Geometry check sheet. Reference: the model listing, model coordinates, mm. A direction names the side the tool comes from. Round coordinates to 2 decimals unless told otherwise and drop trailing zeros. Loops run counter-clockwise (first coordinate to the right, second up) from the corner with the lowest first, then second, coordinate; pieces in that order, holes last.
```python
from build123d import *

# Parameters (mm, degrees)
SKETCH_1_W      = 10
SKETCH_1_H      = 20
SKETCH_1_R      = 1.25
EXTRUDE_1_DEPTH = 1
FILLET_1_R      = 1
SKETCH_13_R     = 0.75


with BuildPart() as part:
    # 草图1 → 凸台-拉伸1 (new body)
    with BuildSketch(Plane.XY):
        with Locations((5, -10)):
            Rectangle(SKETCH_1_W, SKETCH_1_H)
        with Locations((5, -4)):
            Circle(SKETCH_1_R, mode=Mode.SUBTRACT)
        with Locations((5, -16)):
            Circle(SKETCH_1_R, mode=Mode.SUBTRACT)
    extrude(amount=EXTRUDE_1_DEPTH)

    # 圆角1
    fillet_1_edges = [part.edges().sort_by_distance(p)[0] for p in [
        (0, 0, 0.5),
        (10, 0, 0.5),
        (10, -20, 0.5),
        (0, -20, 0.5),
    ]]
    fillet(fillet_1_edges, radius=FILLET_1_R)

    # 扫描11: sweep along a path in 草图5
    with BuildLine(Plane(origin=(0, -10, 0), x_dir=(1, 0, 0), z_dir=(0, 1, 0))) as sweep_11_path:
        Line((1.3, 0), (1.3, 11.5))
        ThreePointArc((1.3, 11.5), (1.739339828, 12.560660172), (2.8, 13))
        Line((2.8, 13), (7.2, 13))
        ThreePointArc((7.2, 13), (8.260660172, 12.560660172), (8.7, 11.5))
        Line((8.7, 11.5), (8.7, 0))
    # 草图13 → 扫描11 (sweep)
    with BuildSketch(Plane(origin=(0, 0, 0), x_dir=(-1, 0, 0), z_dir=(0, 0, -1))):
        with Locations((-8.7, -10)):
            Circle(SKETCH_13_R)
    sweep(path=sweep_11_path.line)


solid = part.part
```
1) Sectioned sample at D-D, the plane z = -0.75. Record the cut outline in (x, y), then the cut area to 3 significant figures.
Report:
outline: circle Ø1.5 at (1.3, -10); circle Ø1.5 at (8.7, -10)
area: 3.53 mm2
2) Sectioned sample at C-C, the plane y = -10. Record the cut outline in (x, z).
Report:
outline: (0, 0) - (0.55, 0) - (0.55, -11.5) arc R2.25 ccw to (2.8, -13.75) - (7.2, -13.75) arc R2.25 ccw to (9.45, -11.5) - (9.45, 0) - (10, 0) - (10, 1) - (0, 1) - close; hole (2.05, -11.5) arc R0.75 ccw to (2.8, -12.25) - (7.2, -12.25) arc R0.75 ccw to (7.95, -11.5) - (7.95, 0) - (2.05, 0) - close
3) Sectioned sample at A-A, the plane y = -4. Record the cut outline in (x, z), then the cut area to 3 significant figures.
Report:
outline: (0, 0) - (3.75, 0) - (3.75, 1) - (0, 1) - close; (6.25, 0) - (10, 0) - (10, 1) - (6.25, 1) - close
area: 7.50 mm2
4) Mould release check, pull along Z, two halves, no side actions. Record for faces 1 (the face through (0.285, -19.699, 0.507)), 2 (the face through (5, -10, 1)), 3 (the face through (5.03, -10.51, -13.55)): +Z half, -Z half, draft (parallel to the pull), parting line (faces both ways), or undercut.
Report:
face 1: draft
face 2: +Z half
face 3: undercut
5) Sectioned sample at B-B, the plane x = 6. Record the cut outline in (y, z).
Report:
outline: (-20, 0) - (-16.75, 0) - (-16.75, 1) - (-20, 1) - close; (-15.25, 0) - (-4.75, 0) - (-4.75, 1) - (-15.25, 1) - close; circle Ø1.5 at (-10, -13); (-3.25, 0) - (0, 0) - (0, 1) - (-3.25, 1) - close
6) Scan lines: line 1 along Y through (x, z) = (5, 0.35); line 2 along Z through (x, y) = (2, -3.25); line 3 along Z through (x, y) = (7.75, -9.5). Record each from-to range of solid material in increasing order.
Report:
line 1: y = -20 to -17.25, -14.75 to -5.25, -2.75 to 0
line 2: z = 0 to 1
line 3: z = -13.48 to -12.26, 0 to 1
7) Access from +Z, -Z, +X, -X, +Y, -Y to the whole of each face (thin tool, end or side, straight path). Record for faces 4 (the face through (1.202, -10.744, -5.83)), 5 (the face through (9.699, -19.715, 0.507)).
Report:
face 4: none
face 5: +Z, -Z, +X, -Y
8) Gauge pin test, flat ends, axial feed: pin 1 (2 mm diameter, centred on x = 5, y = -4, fed in from -Z); pin 2 (3 mm diameter, centred on x = 5, y = -16, fed in from -Z); pin 3 (3 mm diameter, centred on y = -10.5, z = -5.5, fed in from +X). Record the tip position at first contact, or that the pin passes through.
Report:
pin 1: passes through
pin 2: stops at z = 0
pin 3: stops at x = 9.45
